Could you check a few things on this model? Use its own coordinates, in mm. Give positions to 0.01 mm unless a question says otherwise; leave off trailing zeros. Write each loop counter-clockwise with the first axis right and the second up, starting at its lowest first coordinate (ties: lowest second). Pieces come first, ordered by that corner, then holes. Notation, with made-up numbers: M 55.5,42.5 L 98.5,42.5 A24 ccw 98.5,55.5 Z; hole C -15,79.5 d11. An arc over 180 degrees is marked long. One line per item, written item: value.
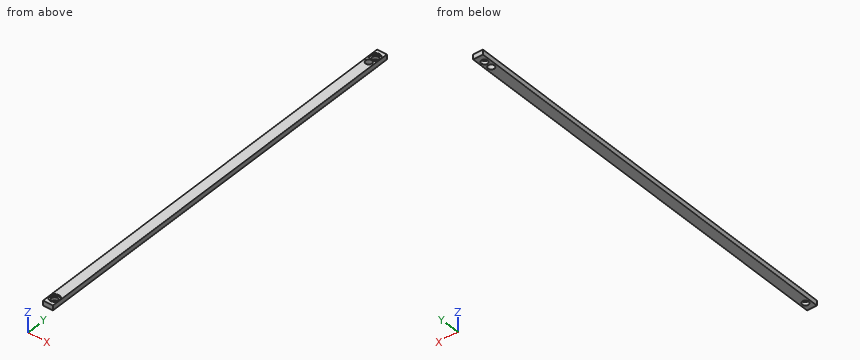
```python
from build123d import *

# Parameters (mm, degrees)
ESQUISSE1_W             = 6
ESQUISSE1_H             = 250
BOSS_EXTRU_1_DEPTH      = 3
ESQUISSE2_R             = 1.95
ENL_V_MAT_EXTRU_1_DEPTH = 3
ESQUISSE3_R             = 2.995
ENL_V_MAT_EXTRU_3_DEPTH = 1


with BuildPart() as part:
    # Esquisse1 → Boss.-Extru.1 (new body)
    with BuildSketch(Plane.XY):
        with Locations((-3, 125)):
            Rectangle(ESQUISSE1_W, ESQUISSE1_H)
    extrude(amount=BOSS_EXTRU_1_DEPTH)

    # Esquisse2 → Enlèv. mat.-Extru.1 (cut)
    with BuildSketch(Plane.XY.offset(3)):
        with Locations((-3, 245)):
            Circle(ESQUISSE2_R)
        with Locations((-3, 240)):
            Circle(ESQUISSE2_R)
        with Locations((-3, 5)):
            Circle(ESQUISSE2_R)
    extrude(amount=-ENL_V_MAT_EXTRU_1_DEPTH, mode=Mode.SUBTRACT)

    # Esquisse3 → Enlèv. mat.-Extru.3 (cut)
    with BuildSketch(Plane.XY.offset(3)):
        with Locations((-3, 5)):
            Circle(ESQUISSE3_R)
        with Locations((-3, 245)):
            Circle(ESQUISSE3_R)
    extrude(amount=-ENL_V_MAT_EXTRU_3_DEPTH, mode=Mode.SUBTRACT)


solid = part.part
```
1) If we section it at B-B, the plane z = 1.5: Write out the boundary of the cut face in (x, y), then the cut area to 3 significant figures.
Outcome:
outline: M -6,0 L 0,0 L 0,250 L -6,250 Z; hole C -3,5 d3.9; hole C -3,240 d3.9; hole C -3,245 d3.9
area: 1,460 mm^2
2) If we section it at A-A, the plane x = -3: Write out the boundary of the cut face in (y, z) (3 decimals), then the cut area to 3 significant figures.
Outcome:
outline: M 0,0 L 3.05,0 L 3.05,2 L 2.005,2 L 2.005,3 L 0,3 Z; M 6.95,0 L 238.05,0 L 238.05,3 L 7.995,3 L 7.995,2 L 6.95,2 Z; M 241.95,0 L 243.05,0 L 243.05,2 L 242.005,2 L 242.005,3 L 241.95,3 Z; M 246.95,0 L 250,0 L 250,3 L 247.995,3 L 247.995,2 L 246.95,2 Z
area: 711 mm^2
3) Please list where these lines run through material, in increasing order: L1, parallel to Y at x = -3, z = 0.9; L2, parallel to X at y = 240, z = 0.8; L3, parallel to Y at x = -1.8, z = 1.1. Write a range as from..to.
Outcome:
L1: y = 0..3.05, 6.95..238.05, 241.95..243.05, 246.95..250
L2: x = -6..-4.95, -1.05..0
L3: y = 0..3.46, 6.54..238.46, 241.54..243.46, 246.54..250
4) I'm going to push flat-ended pins straight in: pin 1 (2.5 mm diameter, centred on x = -3, y = 245, fed in from -Z); pin 2 (1.8 mm diameter, centred on x = -4, y = 6.5, fed in from +Z). Where does each tip first touch, or does it pass through?
Outcome:
pin 1: passes through
pin 2: stops at z = 2
